Can you work these out from the model? Positions are in its coordinate system, mm. A direction names the side the tool comes from. Round coordinates to 2 decimals unless told otherwise and drop trailing zeros. Order: outer loops, then holes, each group sorted by start corner. A loop starts at its lowest first (then second) coordinate and runs counter-clockwise, first axis right, second up. Notation, with made-up numbers: (-3, 22.5) -> (5, 22.5) arc R18 ccw to (5, 27.5) -> close; hole circle Ø7 at (81, 29). An arc over 180 degrees is marked (long way). Use a Markdown table: item, result. Add a question column.
Q1. If we section it at C-C on x = -42: List the corners of the cut face in (y, z) for me (3 decimals).
Q2. For faces 5 (the face through (1.33, 7.65, -3.13)), 6 (the face through (41, -15.875, -3)), 7 (the face through (-9.525, -19, -3)), which set-ups out of +Z, -Z, +X, -X, +Y, -Y let a thin tool reach every point of the face, with its end or its side?
Q3. I need wall thicknesses on line 1 along X through (y, z) = (-4, -3.25); line 2 along X through (y, z) = (-0.5, -5); line 3 along Y through (x, z) = (-15.5, -5.25) (3 decimals). Which ranges of each line are inside material? Lowest first, please. Write a range as [from, to].
Q4. I'm going to push flat-ended pins straight in: pin 1 Ø3 at (y, z) = (12.5, -3.5) entering from +X; pin 2 Ø3 at (x, z) = (-78, -2.5) entering from +Y (3 decimals); pin 3 Ø1 at (x, z) = (-45.5, -2) entering from -Y (3 decimals). Where does each tip first touch, or does it pass through?
Q5. If we section it at A-A on y = -19.05: List the corners of the cut face in (x, z) for me (3 decimals).
Q6. We'd pull the mould along X, two halves only. Please class faces 1 (the face through (-6.35, 5, -3)), 2 (the face through (-73.66, 13, -3)), 3 (the face through (73.66, 13, -3)), 4 (the face through (7.65, -1.33, -3.13)): +X half, -X half, draft (parallel to the pull), parting line (faces both ways), or undercut.
Q7. If we section it at B-B on z = -3: Give the number of separate pieces and of enclosed holes in the cut face, plus the area to 3 significant figures.
```python
from build123d import *

# Parameters (mm, degrees)
SKETCH1_W           = 147.32
SKETCH1_H           = 31.75
BOSS_EXTRUDE1_DEPTH = 6.35
SKETCH2_W           = 6.35
SKETCH2_H           = 19.05
SKETCH2_R           = 1.5
SKETCH2_W_2         = 19.05
SKETCH2_H_2         = 6.35
BOSS_EXTRUDE2_DEPTH = 6.35
CUT_EXTRUDE1_DEPTH  = 6.35


with BuildPart() as part:
    # Sketch1 → Boss-Extrude1 (new body)
    with BuildSketch(Plane.XY):
        Rectangle(SKETCH1_W, SKETCH1_H)
    extrude(amount=-BOSS_EXTRUDE1_DEPTH)

    # Sketch2 → Boss-Extrude2 (add)
    with BuildSketch(Plane.XY):
        with Locations((76.835, 0)):
            Rectangle(SKETCH2_W, SKETCH2_H)
        with Locations((76.835, 0)):
            Circle(SKETCH2_R, mode=Mode.SUBTRACT)
        with Locations((-76.835, 0)):
            Rectangle(SKETCH2_W, SKETCH2_H)
        with Locations((-76.835, 0)):
            Circle(SKETCH2_R, mode=Mode.SUBTRACT)
        with Locations((0, -19.05)):
            Rectangle(SKETCH2_W_2, SKETCH2_H_2)
        with Locations((0, -19.05)):
            Circle(SKETCH2_R, mode=Mode.SUBTRACT)
    extrude(amount=-BOSS_EXTRUDE2_DEPTH)

    # Sketch3 → Cut-Extrude1 (cut)
    with BuildSketch(Plane.XY):
        Polygon((0, -8.980256121), (2.630256121, -6.35), (6.35, -6.35), (6.35, -2.630256121), (8.980256121, 0), (6.35, 2.630256121), (6.35, 6.35), (2.630256121, 6.35), (0, 8.980256121), (-2.630256121, 6.35), (-6.35, 6.35), (-6.35, 2.630256121), (-8.980256121, 0), (-6.35, -2.630256121), (-6.35, -6.35), (-2.630256121, -6.35), align=None)
    extrude(amount=-CUT_EXTRUDE1_DEPTH, mode=Mode.SUBTRACT)


solid = part.part
```
Answer below:
| question | item | result |
|---|---|---|
| 1 | outline | (-15.875, -6.35) -> (15.875, -6.35) -> (15.875, 0) -> (-15.875, 0) -> close |
| 2 | face 5 | +Z, -Z |
| 2 | face 6 | +Z, -Z, +X, -Y |
| 2 | face 7 | +Z, -Z, -X, -Y |
| 3 | line 1 | [-80.01, -6.35], [6.35, 80.01] |
| 3 | line 2 | [-80.01, -78.25], [-75.42, -8.48], [8.48, 75.42], [78.25, 80.01] |
| 3 | line 3 | [-15.875, 15.875] |
| 4 | pin 1 | x = 73.66 |
| 4 | pin 2 | y = 9.525 |
| 4 | pin 3 | y = -15.875 |
| 5 | outline | (-9.525, -6.35) -> (-1.5, -6.35) -> (-1.5, 0) -> (-9.525, 0) -> close; (1.5, -6.35) -> (9.525, -6.35) -> (9.525, 0) -> (1.5, 0) -> close |
| 6 | face 1 | undercut |
| 6 | face 2 | -X half |
| 6 | face 3 | +X half |
| 6 | face 4 | undercut |
| 7 | separate pieces | 1 |
| 7 | enclosed holes | 4 |
| 7 | area | 4,830 mm² |
